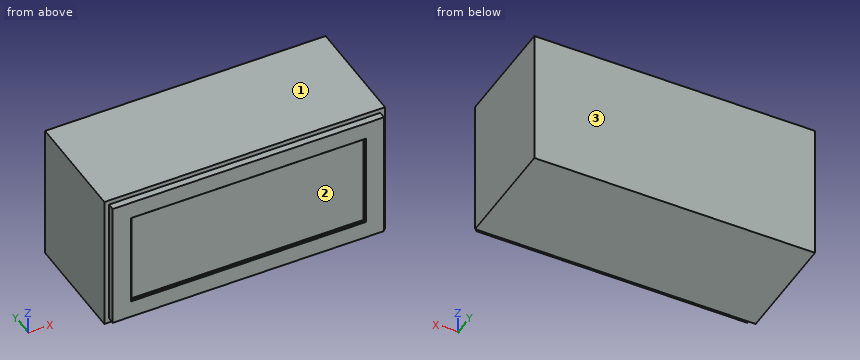
```python
from build123d import *

# Parameters (mm, degrees)
F0_W     = 765.175
F0_H     = 304.8
F1_DEPTH = 381
F2_T     = -12.7
F3_W     = 765.175
F3_H     = 381
F3_W_2   = 749.3
F3_H_2   = 368.3
F3_W_3   = 739.775
F3_H_3   = 355.6
F3_W_4   = 682.625
F3_H_4   = 298.45
F4_DEPTH = 19.05
F3_W_5   = 635
F3_H_5   = 254
F5_DEPTH = 19.05
F6_W     = 7.9375
F6_H     = 254
F7_DEPTH = 635
F8_SIZE  = 3.175


with BuildPart() as f1:
    # F0 (on Top) → F1 (new body)
    with BuildSketch(Plane.XY):
        Rectangle(F0_W, F0_H)
    extrude(amount=F1_DEPTH)

    # F2
    f2_openings = [f1.faces().sort_by_distance(p)[0] for p in [
        (0, -152.4, 190.5),
    ]]
    offset(amount=F2_T, openings=f2_openings)

    # F3 (on face) → F4 (join)
    with BuildSketch(Plane.XZ.offset(152.4)):
        with Locations((0, 190.5)):
            Rectangle(F3_W, F3_H)
        with Locations((0, 190.5)):
            Rectangle(F3_W_2, F3_H_2, mode=Mode.SUBTRACT)
        with Locations((0, 190.5)):
            Rectangle(F3_W_2, F3_H_2)
        with Locations((0, 190.5)):
            Rectangle(F3_W_3, F3_H_3, mode=Mode.SUBTRACT)
        with Locations((0, 190.5)):
            Rectangle(F3_W_3, F3_H_3)
        with Locations((0, 190.5)):
            Rectangle(F3_W_4, F3_H_4, mode=Mode.SUBTRACT)
    extrude(amount=-F4_DEPTH)

    # F3 (on face) → F5 (join)
    with BuildSketch(Plane.XZ.offset(152.4)):
        with Locations((0, 190.5)):
            Rectangle(F3_W_3, F3_H_3)
        with Locations((0, 190.5)):
            Rectangle(F3_W_4, F3_H_4, mode=Mode.SUBTRACT)
        with Locations((0, 190.5)):
            Rectangle(F3_W_4, F3_H_4)
        with Locations((0, 190.5)):
            Rectangle(F3_W_5, F3_H_5, mode=Mode.SUBTRACT)
    extrude(amount=F5_DEPTH)

    # F6 (on face) → F7 (join, through all)
    with BuildSketch(Plane(origin=(317.5, 0, 0), x_dir=(0, -1, 0), z_dir=(-1, 0, 0))):
        with Locations((161.13125, 190.5)):
            Rectangle(F6_W, F6_H)
    extrude(amount=F7_DEPTH)

    # F8
    f8_edges = [f1.edges().sort_by_distance(p)[0] for p in [
        (0, -171.45, 63.5),
        (-317.5, -171.45, 190.5),
        (0, -171.45, 317.5),
        (317.5, -171.45, 190.5),
    ]]
    chamfer(f8_edges, length=F8_SIZE)


solid = f1.part
```
Geometry check sheet. Reference: the model listing, model coordinates, mm. Face numbers are marked on the shaded views. Give positions to 0.01 mm unless a question says otherwise; leave off trailing zeros. Write each loop counter-clockwise with the first axis right and the second up, starting at its lowest first coordinate (ties: lowest second). Pieces come first, ordered by that corner, then holes. Notation, with made-up numbers: (23.5, 29) -> (53.5, 29) arc R23 ccw to (53.5, 37) -> close; hole circle Ø5 at (-24, -38.75). An arc over 180 degrees is marked (long way). One line per question, with ' | ' between items.
Item 1: Sectioned sample at B-B, the plane y = 115. Record the boundary of the cut face in (x, z), plus the area to 3 significant figures.
Determined:
outline: (-382.59, 0) -> (382.59, 0) -> (382.59, 381) -> (-382.59, 381) -> close; hole (-369.89, 12.7) -> (369.89, 12.7) -> (369.89, 368.3) -> (-369.89, 368.3) -> close | area: 28,500 mm^2
Item 2: Scan lines: line 1 along Z through (x, y) = (-269.5, 135); line 2 along X through (y, z) = (127.5, 49.5); line 3 along X through (y, z) = (-147, 284). Record each from-to range of solid material in increasing order.
Determined:
line 1: 0 to 12.7, 368.3 to 381 | line 2: -382.59 to -369.89, 369.89 to 382.59 | line 3: -382.59 to -341.31, 341.31 to 382.59
Item 3: Draft check along Z on the marked faces 1, 2 and 3. Enter one of: released by +Z, released by -Z, zero draft, split by the parting line, or undercut.
Determined:
face 1: released by +Z | face 2: undercut | face 3: zero draft
Item 4: Depth check by flat-ended pin: pin 1 (15 mm diameter, centred on x = 54.5, y = -160.5, fed in from +Z); pin 2 (2.5 mm diameter, centred on x = -79, y = -155, fed in from -Z); pin 3 (15 mm diameter, centred on y = -164, z = 210, fed in from -X). Enter the tip coordinate at first touch or a pass-through.
Determined:
pin 1: z = 368.3 | pin 2: z = 12.7 | pin 3: x = -369.89
